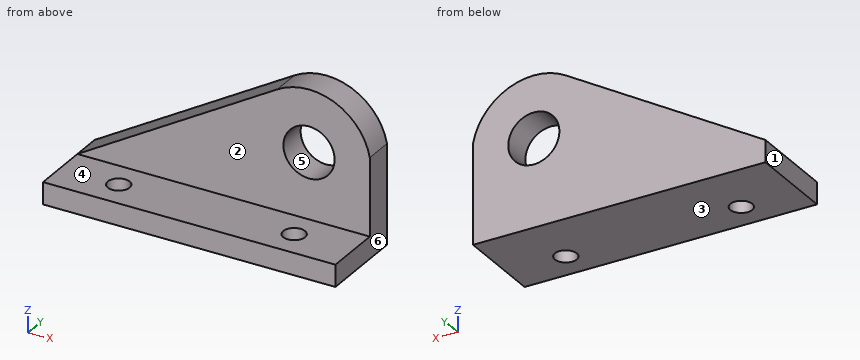
from build123d import *

# Parameters (mm, degrees)
F0_W           = 127
F0_H           = 9.525
F1_DEPTH       = 38.1
F2_DEPTH       = 12.7
F3_D           = 22.225
F3_CBORE_D     = 22.225
F3_CBORE_DEPTH = 22.225
F5_D           = 9.525
F5_CBORE_D     = 9.525
F5_CBORE_DEPTH = 9.525
F6_D           = 9.525
F6_CBORE_D     = 9.525
F6_CBORE_DEPTH = 9.525


with BuildPart() as f1:
    # F0 (on Front) → F1 (new body)
    with BuildSketch(Plane.XZ):
        with Locations((63.5, 4.7625)):
            Rectangle(F0_W, F0_H)
    extrude(amount=F1_DEPTH)

    # F0 (on Front) → F2 (join)
    with BuildSketch(Plane.XZ):
        with BuildLine():
            Line((86.8315583768, 61.2163306665), (0, 9.525))
            Line((0, 9.525), (127, 9.525))
            Line((127, 9.525), (127, 32.9619213127))
            Line((127, 32.9619213127), (127, 43.2380786873))
            ThreePointArc((127, 43.2380786873), (111.5830167561, 62.6551183584), (86.8315583768, 61.2163306665))
        make_face()
    extrude(amount=F2_DEPTH)

    # F3 (through all)
    with Locations(Plane(origin=(0, 0, 0), x_dir=(1, 0, 0), z_dir=(0, 1, 0))):
        with Locations((100.5928441882, -38.1)):
            CounterBoreHole(F3_D / 2, F3_CBORE_D / 2, F3_CBORE_DEPTH)

    # F5 (through all)
    with Locations(Plane.XY.offset(9.525)):
        with Locations((25.4, -25.4)):
            CounterBoreHole(F5_D / 2, F5_CBORE_D / 2, F5_CBORE_DEPTH)

    # F6 (through all)
    with Locations(Plane.XY.offset(9.525)):
        with Locations((101.6, -25.4)):
            CounterBoreHole(F6_D / 2, F6_CBORE_D / 2, F6_CBORE_DEPTH)


solid = f1.part
The listing builds one solid part. Answer for the finished solid, in the listing's coordinates (mm). Face numbers are marked on the shaded views. A direction names the side the tool comes from. Coordinates: 2 decimals unless noted, no trailing zeros. Order: outer loops, then holes, each group sorted by start corner. A loop starts at its lowest first (then second) coordinate and runs counter-clockwise, first axis right, second up. Notation, with made-up numbers: (19.5, 18.25) -> (66.5, 18.25) arc R24 cw to (66.5, 37.25) -> close; hole circle Ø3 at (74.25, 74.5). An arc over 180 degrees is marked (long way). Answer in a Markdown table with one row per item. Add a question column.
Item 1: Find section C-C (x = 101.6). Write down the section's boundary in (y, z) (1 decimal), then the cut area to 3 significant figures.
Item 2: Determine the mould class of the marked faces 3, 4, 5 and 6 for opening direction Z: +Z half, -Z half, draft (parallel to the pull), parting line (faces both ways), or undercut.
Item 3: Find section B-B (z = 38.1). Write down the section's boundary in (x, y), then the cut area to 3 significant figures.
Item 4: Find section A-A (y = -25.4). Write down the section's boundary in (x, z) (1 decimal), then the cut area to 3 significant figures.
Item 5: Which of the six approach directions +Z, -Z, +X, -X, +Y, -Y give full straight-line access (tool end or side, diameter ignored) to the marked faces 1 and 2?
Item 6: Find section D-D (y = -7). Write down the section's boundary in (x, z) (1 decimal).
Item 7: Each of these flat-tipped pins is pushed along its axis until it touches: P1, Ø7.5, axis at x = 52, y = -26, coming from the +Z side (3 decimals); P2, Ø4, axis at x = 96.5, y = -4, coming from the +Z side; P3, Ø2, axis at x = 24, z = 14, coming from the -Y side; P4, Ø3, axis at y = -15, z = 21.5, coming from the -X side. Where does it stop, or does it pass through?
Item 8: Find the intervals of material crossed by L1, parallel to X at y = -25.4, z = 2.25; L2, parallel to X at y = -25, z = 7; L3, parallel to Z at x = 100.5, y = -4, in increasing order. Write a range as from..to.
Result set:
| question | item | result |
|---|---|---|
| 1 | outline | (-38.1, 0) -> (-30.2, 0) -> (-30.2, 9.5) -> (-38.1, 9.5) -> close; (-20.6, 0) -> (0, 0) -> (0, 27) -> (-12.7, 27) -> (-12.7, 9.5) -> (-20.6, 9.5) -> close; (-12.7, 49.2) -> (0, 49.2) -> (0, 65) -> (-12.7, 65) -> close |
| 1 | area | 695 mm² |
| 2 | face 3 | -Z half |
| 2 | face 4 | +Z half |
| 2 | face 5 | undercut |
| 2 | face 6 | draft |
| 3 | outline | (48, -12.7) -> (89.48, -12.7) -> (89.48, 0) -> (48, 0) -> close; (111.71, -12.7) -> (127, -12.7) -> (127, 0) -> (111.71, 0) -> close |
| 3 | area | 721 mm² |
| 4 | outline | (0, 0) -> (20.6, 0) -> (20.6, 9.5) -> (0, 9.5) -> close; (30.2, 0) -> (96.8, 0) -> (96.8, 9.5) -> (30.2, 9.5) -> close; (106.4, 0) -> (127, 0) -> (127, 9.5) -> (106.4, 9.5) -> close |
| 4 | area | 1,030 mm² |
| 5 | face 1 | +Z, -Z, -X, +Y, -Y |
| 5 | face 2 | +Z, +X, -X, -Y |
| 6 | outline | (0, 0) -> (127, 0) -> (127, 43.2) arc R26.9 ccw to (86.8, 61.2) -> (0, 9.5) -> close; hole circle Ø22.2 at (100.6, 38.1) |
| 7 | P1 | stops at z = 9.525 |
| 7 | P2 | stops at z = 64.92 |
| 7 | P3 | stops at y = -12.7 |
| 7 | P4 | passes through |
| 8 | L1 | x = 0..20.64, 30.16..96.84, 106.36..127 |
| 8 | L2 | x = 0..20.65, 30.15..96.85, 106.35..127 |
| 8 | L3 | z = 0..26.99, 49.21..65 |
